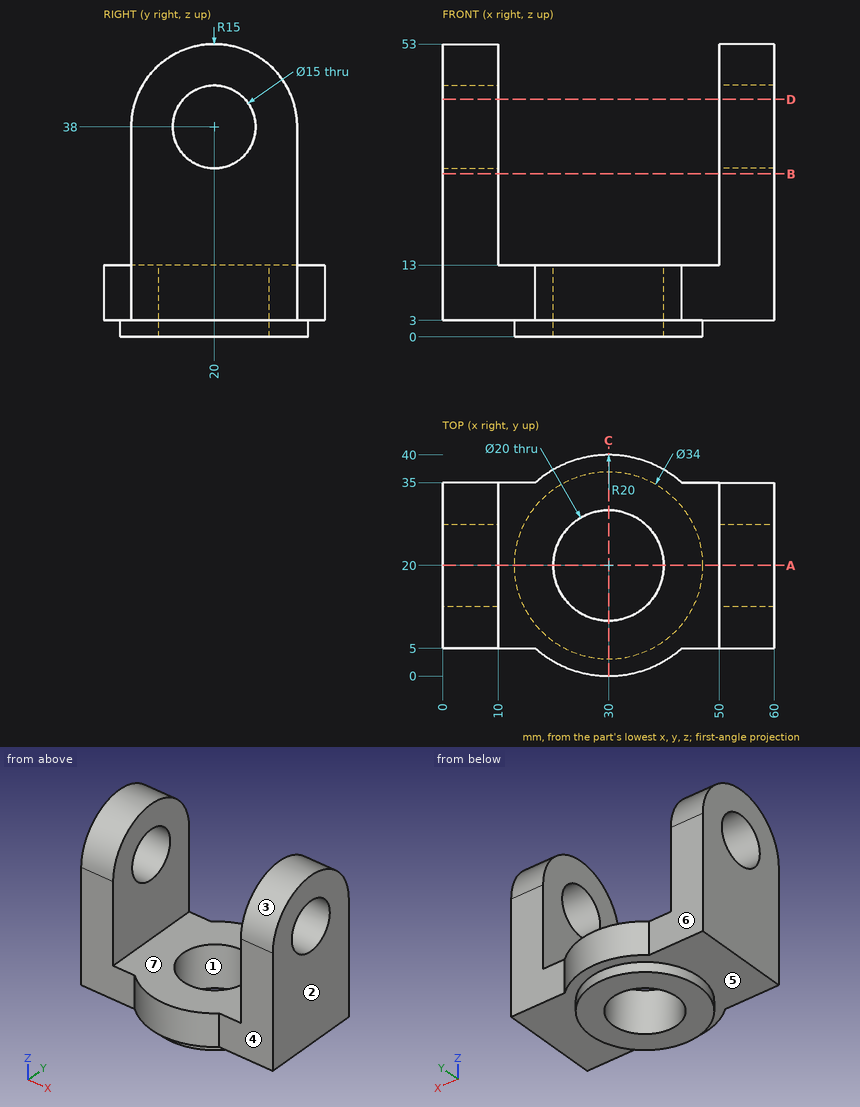
Input: dimensioned drawing with shaded views. Units: mm. Origin: part minimum x, y, z. A direction names the side the tool comes from. Coordinates: 2 decimals unless noted, no trailing zeros. Order: outer loops, then holes, each group sorted by start corner. A loop starts at its lowest first (then second) coordinate and runs counter-clockwise, first axis right, second up.
(1) Section query B-B (z = 29.5). Return the cut outline in (x, y).
(2) Access query for the marked faces 4, 5, 6 and 7. Directions: +Z, -Z, +X, -X, +Y, -Y. A direction counts if a zero-diameter tool reaches every point of the face in a straight line with its end or side. Return the directions, or none.
(3) First-contact query: pin 1 (10 mm diameter, centred on x = 49.5, y = 26, fed in from -Z); pin 2 (10 mm diameter, centred on x = 37, z = 20, fed in from +Y); pin 3 (8.5 mm diameter, centred on x = 52.5, z = 16.5, fed in from -Y); pin 4 (18.5 mm diameter, centred on x = 53.5, z = 22.5, fed in from +Y). Flat tips, straight axial feed; report the tip coordinate or a pass-through.
(4) Section query A-A (y = 20). Return the cut outline in (x, z).
(5) Draft query along Y for the marked faces 1, 2 and 3. Return one class per face: pulls with the +Y half, pulls with the -Y half, needs draft (parallel to the pull), parting line crosses it, or undercut.
(6) Section query D-D (z = 43). Return the cut outline in (x, y).
(7) Section query C-C (x = 30). Return the cut outline in (y, z), plus the area to 3 significant figures.
(8) Material intervals for probe 1 along Z at (x, y) = (5, 20); probe 2 along X at (y, z) = (20, 6.5); probe 3 along X at (y, z) = (7.5, 19), sorted ascending.
Solution:
1. outline: (0, 5) - (10, 5) - (10, 35) - (0, 35) - close; (50, 5) - (60, 5) - (60, 35) - (50, 35) - close
2. face 4: +Z, -Z, +X, -Y
2. face 5: -Z
2. face 6: +Z, -Z, -X, +Y
2. face 7: +Z, +Y, -Y
3. pin 1: stops at z = 0
3. pin 2: passes through
3. pin 3: stops at y = 5
3. pin 4: stops at y = 35
4. outline: (0, 3) - (13, 3) - (13, 0) - (20, 0) - (20, 13) - (10, 13) - (10, 30.5) - (0, 30.5) - close; (0, 45.5) - (10, 45.5) - (10, 53) - (0, 53) - close; (40, 0) - (47, 0) - (47, 3) - (60, 3) - (60, 30.5) - (50, 30.5) - (50, 13) - (40, 13) - close; (50, 45.5) - (60, 45.5) - (60, 53) - (50, 53) - close
5. face 1: undercut
5. face 2: needs draft
5. face 3: parting line crosses it
6. outline: (0, 5.86) - (10, 5.86) - (10, 14.41) - (0, 14.41) - close; (0, 25.59) - (10, 25.59) - (10, 34.14) - (0, 34.14) - close; (50, 5.86) - (60, 5.86) - (60, 14.41) - (50, 14.41) - close; (50, 25.59) - (60, 25.59) - (60, 34.14) - (50, 34.14) - close
7. outline: (0, 3) - (3, 3) - (3, 0) - (10, 0) - (10, 13) - (0, 13) - close; (30, 0) - (37, 0) - (37, 3) - (40, 3) - (40, 13) - (30, 13) - close
7. area: 242 mm2
8. probe 1: z = 3 to 30.5, 45.5 to 53
8. probe 2: x = 0 to 20, 40 to 60
8. probe 3: x = 0 to 10, 50 to 60
